Solid Edge part; units mm, degrees
sketch "Sketch1" plane through (0, 0, 0) normal (0, 0, 1) x (1, 0, 0)
  line L0 (16.5705, -15) -> (27, -15)
  line L1 (39.75, -3) -> (35.75, -3)
  line L2 (39.75, 15) -> (39.75, -3)
  line L3 (39.75, 15) -> (-39.75, 15)
  line L4 (-39.75, 15) -> (-39.75, -3)
  line L5 (-39.75, -3) -> (-35.75, -3)
  line L6 (-27, -15) -> (-16.5705, -15)
  arc A0 (-11.0552, -11) -> (-16.5705, -15) centre (-21.7852, -2.0075) cw
  line L7 (-11.0552, -11) -> (-2.25, -11)
  line L8 (-2.25, -8.75) -> (-2.25, -11)
  line L9 (2.25, -8.75) -> (2.25, -11)
  line L10 (2.25, -11) -> (11.0552, -11)
  arc A1 (16.5705, -15) -> (11.0552, -11) centre (21.7852, -2.0075) cw
  arc A2 (27, -15) -> (35.75, -3) centre (21.7852, -2.0075) ccw
  arc A3 (-35.75, -3) -> (-27, -15) centre (-21.7852, -2.0075) ccw
  arc A4 (-2.25, -8.75) -> (2.25, -8.75) centre (0, -8.75) cw
  circle A5 centre (37.25, 2.5) radius 1
  circle A6 centre (-37.25, 2.5) radius 1
  circle A7 centre (-5.25, -6) radius 1
  circle A8 centre (5.25, -6) radius 1
extrude "Protrusion1" add sketch "Sketch1" along normal blind 1
sketch "Sketch2" plane through (0, 0, 0) normal (0, 0, 1) x (1, 0, 0)
  circle A0 centre (-5.25, -6) radius 1
  circle A1 centre (5.25, -6) radius 1
  circle A2 centre (37.25, 2.5) radius 1
  line L0 (42.75, -3) -> (42.75, 18)
  line L1 (42.75, 18) -> (-42.75, 18)
  line L2 (-42.75, 18) -> (-42.75, -2.0075)
  line L3 (-42.75, -2.4017) -> (-42.75, -2.0075)
  arc A3 (-42.75, -2.4017) -> (-27.1517, -18) centre (-27.1517, -2.4017) ccw
  line L4 (-21.7852, -18) -> (-27.1517, -18)
  line L5 (-21.7852, -18) -> (28.2486, -18)
  arc A4 (28.2486, -18) -> (42.75, -3.4986) centre (28.2486, -3.4986) ccw
  line L6 (42.75, -3.4986) -> (42.75, -3)
  line L7 (44.75, 20) -> (-44.75, 20)
  line L8 (-44.75, 20) -> (-44.75, -2.0075)
  line L9 (-44.75, -2.0075) -> (-44.75, -4.2962)
  arc A5 (-44.75, -4.2962) -> (-29.0462, -20) centre (-29.0462, -4.2962) ccw
  line L10 (-29.0462, -20) -> (-21.7852, -20)
  line L11 (-21.7852, -20) -> (28.0671, -20)
  arc A6 (28.0671, -20) -> (44.75, -3.3171) centre (28.0671, -3.3171) ccw
  line L12 (44.75, -3.3171) -> (44.75, -3)
  line L13 (44.75, -3) -> (44.75, 20)
  circle A7 centre (-37.25, 2.5) radius 1
  circle A8 centre (-5.25, -6) radius 3
  circle A9 centre (-37.25, 2.5) radius 3
  circle A10 centre (5.25, -6) radius 3
  circle A11 centre (37.25, 2.5) radius 3
extrude "ExtrudedProtrusion_2" add sketch "Sketch2" against normal blind 4
sketch "Sketch3" plane through (0, 0, -4) normal (0, 0, -1) x (1, 0, 0)
  line L0 (28.0671, 20) -> (-29.0462, 20)
  arc A0 (-29.0462, 20) -> (-44.75, 4.2962) centre (-29.0462, 4.2962) ccw
  line L1 (-44.75, 4.2962) -> (-44.75, -20)
  line L2 (-44.75, -20) -> (44.75, -20)
  line L3 (44.75, -20) -> (44.75, 3.3171)
  arc A1 (28.0671, 20) -> (44.75, 3.3171) centre (28.0671, 3.3171) cw
extrude "ExtrudedProtrusion_3" add sketch "Sketch3" along normal blind 2
sketch "Sketch4" plane through (0, 0, 0) normal (0, 0, 1) x (1, 0, 0)
  line L0 (-44.75, 20) -> (44.75, 20)
  line L1 (44.75, 20) -> (44.75, -3.3171)
  arc A0 (28.0671, -20) -> (44.75, -3.3171) centre (28.0671, -3.3171) ccw
  line L2 (28.0671, -20) -> (-29.0462, -20)
  arc A1 (-44.75, -4.2962) -> (-29.0462, -20) centre (-29.0462, -4.2962) ccw
  line L3 (-44.75, -4.2962) -> (-44.75, 20)
  line L4 (-42.75, 18) -> (42.75, 18)
  line L5 (42.75, 18) -> (42.75, -3.4986)
  arc A2 (28.2486, -18) -> (42.75, -3.4986) centre (28.2486, -3.4986) ccw
  line L6 (28.2486, -18) -> (-27.1517, -18)
  arc A3 (-42.75, -2.4017) -> (-27.1517, -18) centre (-27.1517, -2.4017) ccw
  line L7 (-42.75, -2.4017) -> (-42.75, 18)
extrude "ExtrudedProtrusion_4" add sketch "Sketch4" along normal blind 14
fillet "Round_1" radius 4 6 edges at (38.5026, -13.7526, -4) (-38.1814, -13.4314, -4) (0.5484, -18, -4) (42.75, 7.2507, -4) (0, 18, -4) (-42.75, 7.7992, -4)
fillet "Round_2" radius 8 5 edges at (-0.4896, -20, -6) (-40.1505, -15.4005, -6) (-44.75, 7.8519, -6) (44.75, 8.3415, -6) (39.8637, -15.1137, -6)
sketch "Sketch5" plane through (0, 0, 14) normal (0, 0, 1) x (1, 0, 0)
  line L0 (-44.75, 20) -> (44.75, 20)
  line L1 (44.75, 20) -> (44.75, -3.3171)
  arc A0 (28.0671, -20) -> (44.75, -3.3171) centre (28.0671, -3.3171) ccw
  line L2 (-29.0462, -20) -> (28.0671, -20)
  arc A1 (-44.75, -4.2962) -> (-29.0462, -20) centre (-29.0462, -4.2962) ccw
  line L3 (-44.75, -4.2962) -> (-44.75, -3.3171)
  line L4 (-44.75, -3.3171) -> (-44.75, 20)
  circle A2 centre (-21.7852, -2.0075) radius 12
  circle A3 centre (21.7852, -2.0075) radius 12
extrude "ExtrudedProtrusion_5" add sketch "Sketch5" along normal blind 2
fillet "Round_5" radius 2 5 edges at (-38.1814, -13.4314, 14) (-42.75, 7.7992, 14) (0.5484, -18, 14) (38.5026, -13.7526, 14) (42.75, 7.2507, 14)
sketch "Sketch6" plane through (0, 0, 1) normal (0, 0, 1) x (0, -1, 0)
  line L0 (37.005, -48.7857) -> (-37.005, -48.7857)
  line L1 (-37.005, -48.7857) -> (-37.005, 48.7857)
  line L2 (-37.005, 48.7857) -> (37.005, 48.7857)
  line L3 (37.005, 48.7857) -> (37.005, -48.7857)
extrude "ExtrudedCutout_2" cut sketch "Sketch6" along normal blind 0.5
sketch "Sketch7" plane through (0, 2, 16) normal (0, 0, 1) x (1, 0, 0)
  line L0 (48.422, -25.3471) -> (-48.422, -25.3471)
  line L1 (-48.422, -25.3471) -> (-48.422, 21.3471)
  line L2 (-48.422, 21.3471) -> (48.422, 21.3471)
  line L3 (48.422, 21.3471) -> (48.422, -25.3471)
extrude "ExtrudedCutout_7" cut sketch "Sketch7" against normal blind 10
sketch "Sketch8" plane through (0, 4, -6) normal (0, 0, -1) x (1, 0, 0)
  line L0 (50.3879, -23.0296) -> (-50.3879, -23.0296)
  line L1 (-50.3879, -23.0296) -> (-50.3879, 31.0296)
  line L2 (-50.3879, 31.0296) -> (50.3879, 31.0296)
  line L3 (50.3879, 31.0296) -> (50.3879, -23.0296)
extrude "Cutout1" cut sketch "Sketch8" against normal up to vertex (8 mm away)
Check sheet for the modelled part. Datum: model origin and axes. Units: mm. A direction names the side the tool comes from. Give positions to 0.01 mm unless a question says otherwise; leave off trailing zeros. Loops run counter-clockwise (first coordinate to the right, second up) from the corner with the lowest first, then second, coordinate; pieces in that order, holes last. Notation, with made-up numbers: (5.25, 52.25) - (21.25, 52.25) arc R16 cw to (21.25, 82.25) - close; hole circle Ø3 at (19.5, 88.25). An arc over 180 degrees is marked (long way). One line per question, with ' | ' between items. Start each with the question number.
1. Material ranges on line 1 along Y through (x, z) = (-11.5, 4); line 2 along X through (y, z) = (2, 5.5); line 3 along X through (y, z) = (-6, 5.65), recorded low to high. Write a range as [from, to].
2. Cross-section at B-B, the plane x = -35. Enter the section's corners in (y, z), plus the area to 3 significant figures.
3. Draft check along X on faces 1 (the cylindrical face through (38.615, -13.639, 3.972)), 2 (the flat face through (1, 20, 4)), 3 (the flat face through (-44.75, 8, 4)), 4 (the cylindrical face through (39.733, -15.243, 4.028)). Enter one of: released by +X, released by -X, zero draft, split by the parting line, or undercut.
4. Cross-section at A-A, the plane z = 3.95. Enter the section's corners in (x, y).
5. Set-up check for faces 5 (the flat face through (0, 19, 2)), 6 (the flat face through (-1, 18, 4)): record each of +Z, -Z, +X, -X, +Y, -Y from which the full face is reachable in a straight line by a thin tool's end or side.
6. Cross-section at C-C, the plane y = 5. Enter the section's corners in (x, z).
Check result:
1) line 1: y = [-20, -18], [18, 20] | line 2: x = [-44.75, -42.75], [42.75, 44.75] | line 3: x = [-44.66, -42.33], [42.53, 44.53]
2) outline: (-18.83, 2) - (-15.88, 2) - (-15.88, 6) - (-18.83, 6) - close; (18, 2) - (20, 2) - (20, 6) - (18, 6) - close | area: 19.8 mm2
3) face 1: undercut | face 2: zero draft | face 3: released by -X | face 4: released by +X
4) outline: (-44.75, -4.3) arc R15.7 ccw to (-29.05, -20) - (28.07, -20) arc R16.68 ccw to (44.75, -3.32) - (44.75, 20) - (-44.75, 20) - close; hole (-42.75, -2.4) arc R15.6 ccw to (-27.15, -18) - (28.25, -18) arc R14.5 ccw to (42.75, -3.5) - (42.75, 18) - (-42.75, 18) - close
5) face 5: -Z, +X, -X, +Y, -Y | face 6: +Z, -Z
6) outline: (-44.75, 2) - (-42.75, 2) - (-42.75, 6) - (-44.75, 6) - close; (42.75, 2) - (44.75, 2) - (44.75, 6) - (42.75, 6) - close
